from build123d import *

# Parameters (mm, degrees)
SKETCH1_R               = 34
BOSS_EXTRUDE1_DEPTH     = 10
SKETCH2_R               = 19.7871926
SKETCH2_R_2             = 2
CUT_EXTRUDE1_DEPTH      = 10
SKETCH3_R               = 4.837531333
SKETCH4_W               = 4.837531333
SKETCH4_H               = 4.837531333
CUT_EXTRUDE3_DEPTH      = 38
CUT_EXTRUDE3_DEPTH_BACK = 38
SKETCH5_W               = 72.361656805
SKETCH5_H               = 8.896778435
BOSS_EXTRUDE2_START     = 60
SKETCH6_R               = 22.2871926
SKETCH6_R_2             = 19.7871926
BOSS_EXTRUDE2_DEPTH     = 60
SKETCH7_R               = 21.0371926
SKETCH7_R_2             = 19.7871926
CUT_EXTRUDE4_DEPTH      = 25
CUT_EXTRUDE6_DEPTH      = 25
CUT_EXTRUDE6_DEPTH_BACK = 25
SKETCH8_R               = 2
CUT_EXTRUDE7_DEPTH      = 43
CUT_EXTRUDE7_DEPTH_BACK = 53
SKETCH9_W               = 69.351432881
SKETCH9_H               = 5.737807944
CUT_EXTRUDE8_START      = -25
SKETCH10_R              = 22.2871926
SKETCH10_R_2            = 21.0371926
CUT_EXTRUDE8_DEPTH      = 25
CUT_EXTRUDE9_DEPTH      = 30
CUT_EXTRUDE9_DEPTH_BACK = 30
SKETCH11_R              = 2


with BuildPart() as part:
    # Sketch1 → Boss-Extrude1 (new body)
    with BuildSketch(Plane(origin=(0, 0, 0), x_dir=(1, 0, 0), z_dir=(0, 1, 0))):
        with Locations(Location((0, 0, 0), (0, 0, 270))):
            Circle(SKETCH1_R)
    extrude(amount=BOSS_EXTRUDE1_DEPTH)

    # Sketch2 → Cut-Extrude1 (cut)
    with BuildSketch(Plane.XZ):
        with Locations(Location((0, 0, 0), (0, 0, 270))):
            Circle(SKETCH2_R)
        with Locations(Location((-22.1, 12.5, 0), (0, 0, 270))):
            Circle(SKETCH2_R_2)
        with Locations(Location((22.1, 12.5, 0), (0, 0, 90))):
            Circle(SKETCH2_R_2)
        with Locations(Location((22.1, -12.5, 0), (0, 0, 270))):
            Circle(SKETCH2_R_2)
        with Locations(Location((-22.1, -12.5, 0), (0, 0, 90))):
            Circle(SKETCH2_R_2)
    extrude(amount=-CUT_EXTRUDE1_DEPTH, mode=Mode.SUBTRACT)

    # Sketch3 → Cut-Revolve1 (revolve, cut)
    with BuildSketch(Plane(origin=(0, 0, 0), x_dir=(0, 0, -1), z_dir=(1, 0, 0)), mode=Mode.PRIVATE) as cut_revolve1_sk:
        with Locations((-34, 5)):
            Circle(SKETCH3_R)
    revolve(cut_revolve1_sk.sketch.rotate(Axis((0, 0, 0), (0, 1, 0)), 180), axis=Axis((0, 0, 0), (0, 1, 0)), mode=Mode.SUBTRACT)

    # Sketch4 → Cut-Revolve2 (revolve, cut)
    with BuildSketch(Plane(origin=(0, 0, 0), x_dir=(0, 0, -1), z_dir=(1, 0, 0)), mode=Mode.PRIVATE) as cut_revolve2_sk:
        with Locations((-31.581234333, 2.581234333)):
            Rectangle(SKETCH4_W, SKETCH4_H)
    revolve(cut_revolve2_sk.sketch.rotate(Axis((0, 0, 0), (0, 1, 0)), 180), axis=Axis((0, 0, 0), (0, 1, 0)), mode=Mode.SUBTRACT)

    # Sketch5 → Cut-Extrude3 (cut, two sides: drawn at the far end of the back side and taken through both)
    with BuildSketch(Plane(origin=(0, 0, 0), x_dir=(0, 0, -1), z_dir=(1, 0, 0)).offset(-CUT_EXTRUDE3_DEPTH_BACK)):
        with Locations((-0.901301775, 0.551610782)):
            Rectangle(SKETCH5_W, SKETCH5_H)
    extrude(amount=CUT_EXTRUDE3_DEPTH + CUT_EXTRUDE3_DEPTH_BACK, mode=Mode.SUBTRACT)

    # Sketch6 → Boss-Extrude2 (add)
    with BuildSketch(Plane.XZ.offset(-5).offset(BOSS_EXTRUDE2_START)):
        with Locations(Location((0, 0, 0), (0, 0, 270))):
            Circle(SKETCH6_R)
        with Locations(Location((0, 0, 0), (0, 0, 270))):
            Circle(SKETCH6_R_2, mode=Mode.SUBTRACT)
    extrude(amount=-BOSS_EXTRUDE2_DEPTH)

    # Sketch7 → Cut-Extrude4 (cut)
    with BuildSketch(Plane.XZ.offset(55)):
        with Locations(Location((0, 0, 0), (0, 0, 270))):
            Circle(SKETCH7_R)
        with Locations(Location((0, 0, 0), (0, 0, 270))):
            Circle(SKETCH7_R_2, mode=Mode.SUBTRACT)
    extrude(amount=-CUT_EXTRUDE4_DEPTH, mode=Mode.SUBTRACT)

    # Sketch8 → Cut-Extrude6 (cut, two sides: drawn at the far end of the back side and taken through both)
    with BuildSketch(Plane(origin=(0, 0, 0), x_dir=(0, 0, -1), z_dir=(1, 0, 0)).offset(-CUT_EXTRUDE6_DEPTH_BACK)):
        with Locations(Location((0, -42.5, 0), (0, 0, 180))):
            Circle(SKETCH8_R)
    extrude(amount=CUT_EXTRUDE6_DEPTH + CUT_EXTRUDE6_DEPTH_BACK, mode=Mode.SUBTRACT)

    # Sketch9 → Cut-Extrude7 (cut, two sides: drawn at the far end of the back side and taken through both)
    with BuildSketch(Plane(origin=(0, 0, 0), x_dir=(0, 0, -1), z_dir=(1, 0, 0)).offset(-CUT_EXTRUDE7_DEPTH_BACK)):
        with Locations((0.165912519, 7.868903972)):
            Rectangle(SKETCH9_W, SKETCH9_H)
    extrude(amount=CUT_EXTRUDE7_DEPTH + CUT_EXTRUDE7_DEPTH_BACK, mode=Mode.SUBTRACT)

    # Sketch10 → Cut-Extrude8 (cut)
    with BuildSketch(Plane(origin=(0, 5, 0), x_dir=(1, 0, 0), z_dir=(0, 1, 0)).offset(CUT_EXTRUDE8_START)):
        with Locations(Location((0, 0, 0), (0, 0, 270))):
            Circle(SKETCH10_R)
        with Locations(Location((0, 0, 0), (0, 0, 90))):
            Circle(SKETCH10_R_2, mode=Mode.SUBTRACT)
    extrude(amount=CUT_EXTRUDE8_DEPTH, mode=Mode.SUBTRACT)

    # Sketch11 → Cut-Extrude9 (cut, two sides: drawn at the far end of the back side and taken through both)
    with BuildSketch(Plane(origin=(0, 0, 0), x_dir=(0, 0, -1), z_dir=(1, 0, 0)).offset(-CUT_EXTRUDE9_DEPTH_BACK)):
        with Locations(Location((0, -7.5, 0), (0, 0, 180))):
            Circle(SKETCH11_R)
    extrude(amount=CUT_EXTRUDE9_DEPTH + CUT_EXTRUDE9_DEPTH_BACK, mode=Mode.SUBTRACT)


solid = part.part
Work out the finished part from the listing and answer in its coordinate system (mm). A direction names the side the tool comes from. Round coordinates to 2 decimals unless told otherwise and drop trailing zeros. Order: outer loops, then holes, each group sorted by start corner. A loop starts at its lowest first (then second) coordinate and runs counter-clockwise, first axis right, second up. Notation, with made-up numbers: M 57,32 L 95,32 A15 cw 95,36 Z; hole C -5.75,-15.75 d5. An arc over 180 degrees is marked long. Put each result on its own line as item: value. Start each with the question number.
Q1. Straight lines are drawn through the part: L1, parallel to Y at x = -20, z = 0; L2, parallel to X at y = -10, z = 0; L3, parallel to X at y = -21, z = 0. For each, find the intervals that lie inside material, in ascending order. Write a range as [from, to].
Q2. For a pull along Y with two mould halves and no side action, classify faces 4 (the flat face through (-19, -30, -8)), 5 (the cylindrical face through (20.4, -6.3, -1.6)), 6 (the flat face through (-8, -20, 20)) as pulls with the +Y half, pulls with the -Y half, needs draft (parallel to the pull), parting line crosses it, or undercut.
Q3. Section C-C, the plane x = 0 is taken. Write down the section's boundary in (y, z).
Q4. A tool of negligible diameter and unlimited length cuts with its end or side. For faces 1 (the cylindrical face through (-20.537, -42.675, 4.56)), 2 (the cylindrical face through (-20.371, -7.588, -1.998)), 3 (the cylindrical face through (20.537, -7.675, 4.56)), from which of +Z, -Z, +X, -X, +Y, -Y can it reach the whole face along a straight path? Write none if from no direction.
Q5. Section B-B, the plane z = 0 is taken. Give the number of separate pieces and of enclosed holes in the cut face, and give its area (3 significant figures).
Q6. Section D-D, the plane z = 16.5 is taken. Write down the section's boundary in (x, y).
Q7. Flat-ended cylindrical pins translate along their axes: pin 1 (2 mm diameter, centred on y = -6.5, z = 7, fed in from +X); pin 2 (8 mm diameter, centred on x = -11.5, z = -7, fed in from +Y); pin 3 (6 mm diameter, centred on x = 2, y = -16.5, fed in from -Z); pin 4 (3 mm diameter, centred on y = -7, z = 15, fed in from -X). Find the tip coordinate at first contact, or state that the pin passes through.
Findings below:
1. L1: y = [-30, -9.5], [-5.5, 5]
1. L2: x = [-21.04, -19.79], [19.79, 21.04]
1. L3: x = [-22.29, -19.79], [19.79, 22.29]
2. face 4: pulls with the -Y half
2. face 5: undercut
2. face 6: pulls with the +Y half
3. outline: M -55,-22.29 L -20,-22.29 L -20,-21.04 L 5,-21.04 L 5,-19.79 L -30,-19.79 L -30,-21.04 L -55,-21.04 Z; M -55,21.04 L -30,21.04 L -30,19.79 L 5,19.79 L 5,21.04 L -20,21.04 L -20,22.29 L -55,22.29 Z
4. face 1: -Y
4. face 2: +X, -X
4. face 3: +Y
5. separate pieces: 6
5. enclosed holes: 0
5. area: 155 mm^2
6. outline: M -14.98,-55 L -13.05,-55 L -13.05,-30 L -10.92,-30 L -10.92,5 L -13.05,5 L -13.05,-20 L -14.98,-20 Z; M 10.92,-30 L 13.05,-30 L 13.05,-55 L 14.98,-55 L 14.98,-20 L 13.05,-20 L 13.05,5 L 10.92,5 Z
7. pin 1: stops at x = 20.16
7. pin 2: passes through
7. pin 3: stops at z = -21.04
7. pin 4: stops at x = -16.13
